```python
from build123d import *

# Parameters (mm, degrees)
F1_DEPTH = 1.5875
F2_R     = 6.35
F3_R     = 12.7


with BuildPart() as f1:
    # F0 (on Front) → F1 (new body, symmetric)
    with BuildSketch(Plane.XZ):
        Polygon((-55.833071, 152.4), (-152.4, 152.4), (-152.4, -152.4), (152.4, -152.4), (152.4, 152.4), (56.139176, 152.4), (35.078053, 184.149631), (-34.771947, 184.149631), align=None)
    extrude(amount=F1_DEPTH, both=True)

    # F2
    f2_edges = [f1.edges().sort_by_distance(p)[0] for p in [
        (152.4, 0, 152.4),
        (-152.4, 0, 152.4),
        (-55.833071, 0, 152.4),
        (-34.771947, 0, 184.149631),
        (35.078053, 0, 184.149631),
        (56.139176, 0, 152.4),
    ]]
    fillet(f2_edges, radius=F2_R)

    # F3
    f3_edges = [f1.edges().sort_by_distance(p)[0] for p in [
        (-152.4, 0, -152.4),
        (152.4, 0, -152.4),
    ]]
    fillet(f3_edges, radius=F3_R)


solid = f1.part
```
Design review of the part built by this model. Coordinates are the model's own, in mm. Give positions to 0.01 mm unless a question says otherwise; leave off trailing zeros. Write each loop counter-clockwise with the first axis right and the second up, starting at its lowest first coordinate (ties: lowest second). Pieces come first, ordered by that corner, then holes. Notation, with made-up numbers: (-13, 76) - (23, 76) arc R13 ccw to (23, 82) - close; hole circle Ø9 at (71, 30.25). An arc over 180 degrees is marked (long way). Return JSON: item names as keys, results as strings. Group by question number.
(1) Mouldability with a two-part tool opening along X and no side actions: class faces 1 (the cylindrical face through (-148.78, -0.02, -148.58)), 2 (the flat face through (45.73, -0.02, 168.09)), 3 (the flat face through (-2, -1.588, 18)) as +X half, -X half, draft (parallel to the pull), parting line (faces both ways), or undercut.
(2) Insertion check: pin 1 (1 mm diameter, centred on x = -90.5, y = -0.5, fed in from +Z). The pin has a flat end and moves straight along its axis. Give the tip position at first contact, or say it passes through.
(3) We need section B-B, the plane x = 94.5. Give the boundary of the cut face in (y, z).
(4) We need section A-A, the plane y = 0.05. Give the boundary of the cut face in (x, z).
(5) We need section C-C, the plane z = 160.5. Give the boundary of the cut face in (x, y).
(6) To check wall thickness, follow probe 1 along Z at (x, y) = (-105, -0.75); probe 2 along Z at (x, y) = (-33, -0.45); probe 3 along X at (y, z) = (0.3, 163). State the ranges of each line that lie inside material, in increasing order.
Reported:
{
 "1": {"face 1": "-X half", "face 2": "+X half", "face 3": "draft"},
 "2": {"pin 1": "stops at z = 152.4"},
 "3": {"outline": "(-1.59, -152.4) - (1.59, -152.4) - (1.59, 152.4) - (-1.59, 152.4) - close"},
 "4": {"outline": "(-152.4, -139.7) arc R12.7 ccw to (-139.7, -152.4) - (139.7, -152.4) arc R12.7 ccw to (152.4, -139.7) - (152.4, 146.05) arc R6.35 ccw to (146.05, 152.4) - (59.55, 152.4) arc R6.35 cw to (54.26, 155.24) - (36.96, 181.31) arc R6.35 ccw to (31.67, 184.15) - (-31.36, 184.15) arc R6.35 ccw to (-36.66, 181.31) - (-53.95, 155.24) arc R6.35 cw to (-59.24, 152.4) - (-146.05, 152.4) arc R6.35 ccw to (-152.4, 146.05) - close"},
 "5": {"outline": "(-50.46, -1.59) - (50.77, -1.59) - (50.77, 1.59) - (-50.46, 1.59) - close"},
 "6": {"probe 1": "z = -152.4 to 152.4", "probe 2": "z = -152.4 to 183.94", "probe 3": "x = -48.8 to 49.11"}
}
